```python
from build123d import *

# Parameters (mm, degrees)
SKETCH1_W           = 90
SKETCH1_H           = 115
BOSS_EXTRUDE1_DEPTH = 5
FILLET4_R           = 5
FILLET5_R           = 5
FILLET6_R           = 5
FILLET7_R           = 5
SKETCH4_W           = 25.5
SKETCH4_H           = 5
BOSS_EXTRUDE2_DEPTH = 5
FILLET12_R          = 2.5
FILLET13_R          = 2.5
SKETCH7_R           = 1.27
CUT_EXTRUDE2_DEPTH  = 74.186405842


with BuildPart() as part:
    # Sketch1 → Boss-Extrude1 (new body)
    with BuildSketch(Plane(origin=(0, 0, 0), x_dir=(1, 0, 0), z_dir=(0, 1, 0))):
        Rectangle(SKETCH1_W, SKETCH1_H)
    extrude(amount=BOSS_EXTRUDE1_DEPTH)

    # Fillet4
    fillet4_edges = [part.edges().sort_by_distance(p)[0] for p in [
        (0, 5, 57.5),
    ]]
    fillet(fillet4_edges, radius=FILLET4_R - 0.0001)  # a hair under: the kernel refuses the full size

    # Fillet5
    fillet5_edges = [part.edges().sort_by_distance(p)[0] for p in [
        (-45, 5, -2.49995),
        (-45, 3.535563195, 56.035563195),
    ]]
    fillet(fillet5_edges, radius=FILLET5_R - 0.0001)  # a hair under: the kernel refuses the full size

    # Fillet6
    fillet6_edges = [part.edges().sort_by_distance(p)[0] for p in [
        (45, 5, -2.49995),
        (45, 3.535563195, 56.035563195),
    ]]
    fillet(fillet6_edges, radius=FILLET6_R - 0.0001)  # a hair under: the kernel refuses the full size

    # Fillet7
    fillet7_edges = [part.edges().sort_by_distance(p)[0] for p in [
        (-43.535563195, 3.535563195, -57.5),
        (0, 5, -57.5),
        (43.535563195, 3.535563195, -57.5),
    ]]
    fillet(fillet7_edges, radius=FILLET7_R - 0.0001)  # a hair under: the kernel refuses the full size

    # Sketch4 → Boss-Extrude2 (add)
    with BuildSketch(Plane.XZ):
        with Locations((27.25, 33.466653617)):
            Rectangle(SKETCH4_W, SKETCH4_H)
    extrude(amount=BOSS_EXTRUDE2_DEPTH)

    # Fillet12
    fillet12_edges = [part.edges().sort_by_distance(p)[0] for p in [
        (27.25, -5, 35.966653617),
    ]]
    fillet(fillet12_edges, radius=FILLET12_R)

    # Fillet13
    fillet13_edges = [part.edges().sort_by_distance(p)[0] for p in [
        (27.25, -5, 30.966653617),
    ]]
    fillet(fillet13_edges, radius=FILLET13_R - 0.0001)  # a hair under: the kernel refuses the full size

    # Sketch7 → Cut-Extrude2 (cut, through all)
    with BuildSketch(Plane.XZ):
        with Locations(Location((-40, -52.5, 0), (0, 0, 270))):
            Circle(SKETCH7_R)
        with Locations(Location((40.003969698, -52.469833039, 0), (0, 0, 270))):
            Circle(SKETCH7_R)
        with Locations(Location((39.961684065, 52.494524109, 0), (0, 0, 270))):
            Circle(SKETCH7_R)
        with Locations(Location((-39.980749964, 52.482200306, 0), (0, 0, 270))):
            Circle(SKETCH7_R)
    extrude(amount=-CUT_EXTRUDE2_DEPTH, mode=Mode.SUBTRACT)


solid = part.part
```
Geometry check sheet. Reference: the model listing, model coordinates, mm. A direction names the side the tool comes from. Give positions to 0.01 mm unless a question says otherwise; leave off trailing zeros. Use one line per item in the form item = value.
Item 1: Mould release check, pull along X, two halves, no side actions. Record for faces 1 (the flat face through (40, -2, 33)), 2 (the cylindrical face through (27.4, -4.2, 35.3)), 3 (the cylindrical face through (41.22, 2.47, 52.66)), 4 (the cylindrical face through (38.9, 2.5, -53.1)): released by +X, released by -X, zero draft, split by the parting line, or undercut.
Results list:
face_1 = released by +X
face_2 = zero draft
face_3 = undercut
face_4 = undercut
Item 2: Access from +Z, -Z, +X, -X, +Y, -Y to the whole of each face (thin tool, end or side, straight path). Record for faces 5 (the flat face through (14.5, -2, 33)), 6 (the flat face through (27, -1, 35.967)), 7 (the flat face through (27, -1, 30.967)).
Results list:
face_5 = +Z, -Z, -X, -Y
face_6 = +Z, +X, -X, -Y
face_7 = -Z, +X, -X, -Y
Item 3: Scan lines: line 1 (X direction, y = 4, z = 52); line 2 (X direction, y = 1.1, z = -52.5); line 3 (Y direction, x = -12, z = -46). Record each from-to range of solid material in increasing order.
Results list:
line_1 = -43 to -41.16, -38.81 to 38.79, 41.13 to 43
line_2 = -44.88 to -41.27, -38.73 to 38.73, 41.27 to 44.88
line_3 = 0 to 5
Item 4: Depth check by flat-ended pin: pin 1 Ø2.5 at (y, z) = (-3, 33.5) entering from -X; pin 2 Ø8 at (x, z) = (14.5, 3) entering from -Y; pin 3 Ø0.8 at (x, y) = (28.5, -1.5) entering from -Z. Enter the tip coordinate at first touch or a pass-through.
Results list:
pin_1 = 14.5
pin_2 = 0
pin_3 = 30.97
